Geometry check sheet. Reference: the model listing, model coordinates, mm. Give positions to 0.01 mm unless a question says otherwise; leave off trailing zeros. Loops run counter-clockwise (first coordinate to the right, second up) from the corner with the lowest first, then second, coordinate; pieces in that order, holes last. Notation, with made-up numbers: (84, 88.5) -> (111, 88.5) arc R14 cw to (111, 92.5) -> close; hole circle Ø11 at (-10, 55). An arc over 180 degrees is marked (long way). One line per item, written item: value. Start each with the question number.
(1) Draft check along Y on faces 1 (the face through (351, 103, 3.175)), 2 (the face through (396.946, 95.286, 1.61)). Enter one of: pulls with the +Y half, pulls with the -Y half, needs draft (parallel to the pull), parting line crosses it, or undercut.
(2) Sectioned sample at B-B, the plane z = 2.25. State how many separate pieces and enclosed holes the cut face has, then the cut area to 3 significant figures.
(3) Scan lines: line 1 along Y through (x, z) = (698.5, 2.25); line 2 along Y through (x, z) = (622.3, 1.75); line 3 along X through (y, z) = (120, 2.3). Record each from-to range of solid material in increasing order. Write a range as from..to.
(4) Gauge pin test, flat ends, axial feed: pin 1 Ø3 at (x, y) = (292, 36) entering from -Z; pin 2 Ø3 at (x, y) = (622.3, 190.5) entering from +Z. Record the tip position at first contact, or that the pin passes through.
(5) Sectioned sample at C-C, the plane y = 25. Record the cut outline in (x, z) (3 decimals), then the cut area to 3 significant figures.
(6) Sectioned sample at A-A, the plane y = 123.5. Record the cut outline in (x, z) (3 decimals).
from build123d import *

# Parameters (mm, degrees)
SKETCH1_W           = 711.2
SKETCH1_H           = 203.2
BOSS_EXTRUDE1_DEPTH = 3.175
CUT_EXTRUDE1_REACH  = 5.175
SKETCH2_R           = 2.413
CUT_EXTRUDE2_REACH  = 5.175
SKETCH3_R           = 73.025


with BuildPart() as part:
    # Sketch1 → Boss-Extrude1 (new body)
    with BuildSketch(Plane.XY):
        with Locations((355.6, 101.6)):
            Rectangle(SKETCH1_W, SKETCH1_H)
    extrude(amount=BOSS_EXTRUDE1_DEPTH)

    # Sketch2 → Cut-Extrude1 (cut, up to next)
    with BuildSketch(Plane.XY.offset(3.175), mode=Mode.PRIVATE) as cut_extrude1_sk1:
        with Locations((12.7, 114.3)):
            Circle(SKETCH2_R)
    cut_extrude1_tool1 = extrude(cut_extrude1_sk1.sketch, amount=-CUT_EXTRUDE1_REACH, mode=Mode.PRIVATE) & part.part
    add(cut_extrude1_tool1.solids().sort_by_distance((12.7, 114.3, 3.175))[0], mode=Mode.SUBTRACT)
    # Sketch2 → Cut-Extrude1 (cut, up to next)
    with BuildSketch(Plane.XY.offset(3.175), mode=Mode.PRIVATE) as cut_extrude1_sk2:
        with Locations((698.5, 114.3)):
            Circle(SKETCH2_R)
    cut_extrude1_tool2 = extrude(cut_extrude1_sk2.sketch, amount=-CUT_EXTRUDE1_REACH, mode=Mode.PRIVATE) & part.part
    add(cut_extrude1_tool2.solids().sort_by_distance((698.5, 114.3, 3.175))[0], mode=Mode.SUBTRACT)
    # Sketch2 → Cut-Extrude1 (cut, up to next)
    with BuildSketch(Plane.XY.offset(3.175), mode=Mode.PRIVATE) as cut_extrude1_sk3:
        with Locations((12.7, 38.1)):
            Circle(SKETCH2_R)
    cut_extrude1_tool3 = extrude(cut_extrude1_sk3.sketch, amount=-CUT_EXTRUDE1_REACH, mode=Mode.PRIVATE) & part.part
    add(cut_extrude1_tool3.solids().sort_by_distance((12.7, 38.1, 3.175))[0], mode=Mode.SUBTRACT)
    # Sketch2 → Cut-Extrude1 (cut, up to next)
    with BuildSketch(Plane.XY.offset(3.175), mode=Mode.PRIVATE) as cut_extrude1_sk4:
        with Locations((698.5, 38.1)):
            Circle(SKETCH2_R)
    cut_extrude1_tool4 = extrude(cut_extrude1_sk4.sketch, amount=-CUT_EXTRUDE1_REACH, mode=Mode.PRIVATE) & part.part
    add(cut_extrude1_tool4.solids().sort_by_distance((698.5, 38.1, 3.175))[0], mode=Mode.SUBTRACT)
    # Sketch2 → Cut-Extrude1 (cut, up to next)
    with BuildSketch(Plane.XY.offset(3.175), mode=Mode.PRIVATE) as cut_extrude1_sk5:
        with Locations((88.9, 190.5)):
            Circle(SKETCH2_R)
    cut_extrude1_tool5 = extrude(cut_extrude1_sk5.sketch, amount=-CUT_EXTRUDE1_REACH, mode=Mode.PRIVATE) & part.part
    add(cut_extrude1_tool5.solids().sort_by_distance((88.9, 190.5, 3.175))[0], mode=Mode.SUBTRACT)
    # Sketch2 → Cut-Extrude1 (cut, up to next)
    with BuildSketch(Plane.XY.offset(3.175), mode=Mode.PRIVATE) as cut_extrude1_sk6:
        with Locations((165.1, 190.5)):
            Circle(SKETCH2_R)
    cut_extrude1_tool6 = extrude(cut_extrude1_sk6.sketch, amount=-CUT_EXTRUDE1_REACH, mode=Mode.PRIVATE) & part.part
    add(cut_extrude1_tool6.solids().sort_by_distance((165.1, 190.5, 3.175))[0], mode=Mode.SUBTRACT)
    # Sketch2 → Cut-Extrude1 (cut, up to next)
    with BuildSketch(Plane.XY.offset(3.175), mode=Mode.PRIVATE) as cut_extrude1_sk7:
        with Locations((241.3, 190.5)):
            Circle(SKETCH2_R)
    cut_extrude1_tool7 = extrude(cut_extrude1_sk7.sketch, amount=-CUT_EXTRUDE1_REACH, mode=Mode.PRIVATE) & part.part
    add(cut_extrude1_tool7.solids().sort_by_distance((241.3, 190.5, 3.175))[0], mode=Mode.SUBTRACT)
    # Sketch2 → Cut-Extrude1 (cut, up to next)
    with BuildSketch(Plane.XY.offset(3.175), mode=Mode.PRIVATE) as cut_extrude1_sk8:
        with Locations((622.3, 190.5)):
            Circle(SKETCH2_R)
    cut_extrude1_tool8 = extrude(cut_extrude1_sk8.sketch, amount=-CUT_EXTRUDE1_REACH, mode=Mode.PRIVATE) & part.part
    add(cut_extrude1_tool8.solids().sort_by_distance((622.3, 190.5, 3.175))[0], mode=Mode.SUBTRACT)
    # Sketch2 → Cut-Extrude1 (cut, up to next)
    with BuildSketch(Plane.XY.offset(3.175), mode=Mode.PRIVATE) as cut_extrude1_sk9:
        with Locations((546.1, 190.5)):
            Circle(SKETCH2_R)
    cut_extrude1_tool9 = extrude(cut_extrude1_sk9.sketch, amount=-CUT_EXTRUDE1_REACH, mode=Mode.PRIVATE) & part.part
    add(cut_extrude1_tool9.solids().sort_by_distance((546.1, 190.5, 3.175))[0], mode=Mode.SUBTRACT)
    # Sketch2 → Cut-Extrude1 (cut, up to next)
    with BuildSketch(Plane.XY.offset(3.175), mode=Mode.PRIVATE) as cut_extrude1_sk10:
        with Locations((469.9, 190.5)):
            Circle(SKETCH2_R)
    cut_extrude1_tool10 = extrude(cut_extrude1_sk10.sketch, amount=-CUT_EXTRUDE1_REACH, mode=Mode.PRIVATE) & part.part
    add(cut_extrude1_tool10.solids().sort_by_distance((469.9, 190.5, 3.175))[0], mode=Mode.SUBTRACT)
    # Sketch2 → Cut-Extrude1 (cut, up to next)
    with BuildSketch(Plane.XY.offset(3.175), mode=Mode.PRIVATE) as cut_extrude1_sk11:
        with Locations((393.7, 190.5)):
            Circle(SKETCH2_R)
    cut_extrude1_tool11 = extrude(cut_extrude1_sk11.sketch, amount=-CUT_EXTRUDE1_REACH, mode=Mode.PRIVATE) & part.part
    add(cut_extrude1_tool11.solids().sort_by_distance((393.7, 190.5, 3.175))[0], mode=Mode.SUBTRACT)
    # Sketch2 → Cut-Extrude1 (cut, up to next)
    with BuildSketch(Plane.XY.offset(3.175), mode=Mode.PRIVATE) as cut_extrude1_sk12:
        with Locations((317.5, 190.5)):
            Circle(SKETCH2_R)
    cut_extrude1_tool12 = extrude(cut_extrude1_sk12.sketch, amount=-CUT_EXTRUDE1_REACH, mode=Mode.PRIVATE) & part.part
    add(cut_extrude1_tool12.solids().sort_by_distance((317.5, 190.5, 3.175))[0], mode=Mode.SUBTRACT)

    # Sketch3 → Cut-Extrude2 (cut, up to next)
    with BuildSketch(Plane.XY.offset(3.175), mode=Mode.PRIVATE) as cut_extrude2_sk1:
        with Locations((469.9, 92.075)):
            Circle(SKETCH3_R)
    cut_extrude2_tool1 = extrude(cut_extrude2_sk1.sketch, amount=-CUT_EXTRUDE2_REACH, mode=Mode.PRIVATE) & part.part
    add(cut_extrude2_tool1.solids().sort_by_distance((469.9, 92.075, 3.175))[0], mode=Mode.SUBTRACT)


solid = part.part
Calculated:
1. face 1: needs draft
1. face 2: undercut
2. separate pieces: 1
2. enclosed holes: 13
2. area: 128,000 mm2
3. line 1: y = 0..35.69, 40.51..111.89, 116.71..203.2
3. line 2: y = 0..188.09, 192.91..203.2
3. line 3: x = 0..402.43, 537.37..711.2
4. pin 1: stops at z = 0
4. pin 2: passes through
5. outline: (0, 0) -> (441.028, 0) -> (441.028, 3.175) -> (0, 3.175) -> close; (498.772, 0) -> (711.2, 0) -> (711.2, 3.175) -> (498.772, 3.175) -> close
5. area: 2,070 mm2
6. outline: (0, 0) -> (403.982, 0) -> (403.982, 3.175) -> (0, 3.175) -> close; (535.818, 0) -> (711.2, 0) -> (711.2, 3.175) -> (535.818, 3.175) -> close
